```python
from build123d import *

# Parameters (mm, degrees)
F0_W     = 50.8
F0_H     = 50.8
F0_R     = 12.7
F1_DEPTH = 50.8
F2_R     = 12.7
F3_DEPTH = 25.4
F4_R     = 12.7
F5_DEPTH = 25.4


with BuildPart() as f1:
    # F0 (on Top) → F1 (new body)
    with BuildSketch(Plane.XY):
        Rectangle(F0_W, F0_H)
        Circle(F0_R, mode=Mode.SUBTRACT)
    extrude(amount=F1_DEPTH)

    # F2 (on face) → F3 (cut)
    with BuildSketch(Plane.XZ.offset(25.4)):
        with Locations((0, 23.192675)):
            Circle(F2_R)
    extrude(amount=-F3_DEPTH, mode=Mode.SUBTRACT)

    # F4 (on face) → F5 (join)
    with BuildSketch(Plane.YZ.offset(25.4)):
        with Locations((0, 25.4)):
            Circle(F4_R)
    extrude(amount=F5_DEPTH)


solid = f1.part
```
Input: part model. Units: mm. Frame: model coordinates. A direction names the side the tool comes from. Round coordinates to 2 decimals unless told otherwise and drop trailing zeros. Loops run counter-clockwise (first coordinate to the right, second up) from the corner with the lowest first, then second, coordinate; pieces in that order, holes last. Notation, with made-up numbers: M -31,12.25 L -16,12.25 A22 cw -16,50.25 Z; hole C 77.5,-20.5 d2. An arc over 180 degrees is marked long. Answer in a Markdown table with one row per item. Add a question column.
1. Section A-A (x = 0). Output: boundary loops of the cut face in (y, z), and give its area (3 significant figures).
2. Section B-B (y = -10). Output: boundary loops of the cut face in (x, z).
3. Section D-D (y = 8.5). Output: boundary loops of the cut face in (x, z).
4. Mould query, pull axis Y, two halves, no side actions, for faces 4 (the face through (0, 25.4, 25)), 5 (the face through (25.4, -6, 14)), 6 (the face through (-1.653, 12.592, 25.044)), 7 (the face through (-0.4, -25.4, 36.3)). Classes: released by +Y, released by -Y, zero draft, split by the parting line, or undercut.
5. Section C-C (z = 8). Output: boundary loops of the cut face in (x, y), and give its area (3 significant figures).
6. Contact query for flat-ended pins moving along their axis: pin 1 (3 mm diameter, centred on x = 26, y = -17.5, fed in from -Z); pin 2 (2 mm diameter, centred on x = 39, z = 15.5, fed in from -Y); pin 3 (2 mm diameter, centred on y = 2, z = 40, fed in from +X); pin 4 (20.5 mm diameter, centred on x = 0, y = 0, fed in from +Z). Output: stop coordinate, or through.
7. Ray query, probe 1 along X at (y, z) = (0, 16); probe 2 along X at (y, z) = (-23, 22.5); probe 3 along X at (y, z) = (-14, 39.5). Return the intervals inside material, ascending.
8. Set-up query: faces 1 (the face through (37.922, 6.827, 36.109)), 2 (the face through (50.8, 0, 26)), 3 (the face through (-9.36, -15.7, 31.776)). Return all of +Z, -Z, +X, -X, +Y, -Y with unobstructed straight access to the full face (end or side cutting, diameter ignored); none if empty.
Values follow:
| question | item | result |
|---|---|---|
| 1 | outline | M -25.4,0 L -12.7,0 L -12.7,10.49 L -25.4,10.49 Z; M -25.4,35.89 L -12.7,35.89 L -12.7,50.8 L -25.4,50.8 Z; M 12.7,0 L 25.4,0 L 25.4,50.8 L 12.7,50.8 Z |
| 1 | area | 968 mm^2 |
| 2 | outline | M -25.4,0 L -7.83,0 L -7.83,13.19 A12.7 cw -7.83,33.19 L -7.83,50.8 L -25.4,50.8 Z; M 7.83,0 L 25.4,0 L 25.4,17.57 L 50.8,17.57 L 50.8,33.23 L 25.4,33.23 L 25.4,50.8 L 7.83,50.8 L 7.83,33.19 A12.7 cw 7.83,13.19 Z |
| 3 | outline | M -25.4,0 L -9.44,0 L -9.44,50.8 L -25.4,50.8 Z; M 9.44,0 L 25.4,0 L 25.4,15.96 L 50.8,15.96 L 50.8,34.84 L 25.4,34.84 L 25.4,50.8 L 9.44,50.8 Z |
| 4 | face 4 | released by +Y |
| 4 | face 5 | zero draft |
| 4 | face 6 | undercut |
| 4 | face 7 | released by -Y |
| 5 | outline | M -25.4,-25.4 L 25.4,-25.4 L 25.4,25.4 L -25.4,25.4 Z; hole C 0,0 d25.4 |
| 5 | area | 2,070 mm^2 |
| 6 | pin 1 | z = 0 |
| 6 | pin 2 | y = -9.06 |
| 6 | pin 3 | x = 25.4 |
| 6 | pin 4 | through |
| 7 | probe 1 | -25.4 to -12.7, 12.7 to 50.8 |
| 7 | probe 2 | -25.4 to -12.68, 12.68 to 25.4 |
| 7 | probe 3 | -25.4 to 25.4 |
| 8 | face 1 | +X |
| 8 | face 2 | +Z, -Z, +X, +Y, -Y |
| 8 | face 3 | -Y |
